```python
from build123d import *

# Parameters (mm, degrees)
SKETCH_1_W          = 33
SKETCH_1_H          = 10
EXTRUDE_1_DEPTH     = 3
HOLE_WIZARD_1_D     = 3.5
SKETCH_5_W          = 33
SKETCH_5_H          = 3
EXTRUDE_2_DEPTH     = 3
SKETCH_6_W          = 33
SKETCH_6_H          = 4
EXTRUDE_3_DEPTH     = 55
SKETCH_7_W          = 50
SKETCH_7_H          = 4
EXTRUDE_4_DEPTH     = 3
SKETCH_8_W          = 50
SKETCH_8_H          = 3
EXTRUDE_5_DEPTH     = 56
EXTRUDE_6_DEPTH     = 5
EXTRUDE_7_DEPTH     = 4
SKETCH_20_W         = 50
SKETCH_20_H         = 3
EXTRUDE_9_DEPTH     = 40
EXTRUDE_15_DEPTH    = 4
EXTRUDE_16_DEPTH    = 4
FILLET_1_R          = 3
HOLE_WIZARD_5_D     = 3.5
HOLE_WIZARD_6_D     = 34
HOLE_WIZARD_7_D     = 2.3
EXTRUDE_17_DEPTH    = 5
SKETCH_49_W         = 44.612037216
SKETCH_49_H         = 28
EXTRUDE_18_DEPTH    = 5
SKETCH_50_W         = 11.25
SKETCH_50_H         = 12
CUT_EXTRUDE_1_DEPTH = 10
EXTRUDE_19_DEPTH    = 5
FILLET_2_R          = 5
SKETCH_52_W         = 3
SKETCH_52_H         = 12
CUT_EXTRUDE_2_DEPTH = 126.136925006
FILLET_3_R          = 3
FILLET_4_R          = 5
SKETCH_53_W         = 5
SKETCH_53_H         = 55.387962784
SKETCH_53_H_2       = 45
EXTRUDE_20_DEPTH    = 4


with BuildPart() as part:
    # 草图1 → 凸台-拉伸1 (new body)
    with BuildSketch(Plane(origin=(0, 0, 0), x_dir=(1, 0, 0), z_dir=(0, 1, 0))):
        Rectangle(SKETCH_1_W, SKETCH_1_H)
    extrude(amount=EXTRUDE_1_DEPTH)

    # 孔1 (through all)
    with Locations(Plane(origin=(0, 3, 0), x_dir=(1, 0, 0), z_dir=(0, 1, 0))):
        with Locations((-13, -1.5), (13, -1.5)):
            Hole(HOLE_WIZARD_1_D / 2)

    # 草图5 → 凸台-拉伸2 (add)
    with BuildSketch(Plane.XZ):
        with Locations((0, -6.5)):
            Rectangle(SKETCH_5_W, SKETCH_5_H)
    extrude(amount=-EXTRUDE_2_DEPTH)

    # 草图6 → 凸台-拉伸3 (add)
    with BuildSketch(Plane(origin=(0, 3, 0), x_dir=(1, 0, 0), z_dir=(0, 1, 0))):
        with Locations((0, 6)):
            Rectangle(SKETCH_6_W, SKETCH_6_H)
    extrude(amount=EXTRUDE_3_DEPTH)

    # 草图7 → 凸台-拉伸4 (add)
    with BuildSketch(Plane(origin=(0, 58, 0), x_dir=(1, 0, 0), z_dir=(0, 1, 0))):
        with Locations((-8.5, 6)):
            Rectangle(SKETCH_7_W, SKETCH_7_H)
    extrude(amount=EXTRUDE_4_DEPTH)

    # 草图8 → 凸台-拉伸5 (add)
    with BuildSketch(Plane(origin=(0, 0, -8), x_dir=(-1, 0, 0), z_dir=(0, 0, -1))):
        with Locations((8.5, 59.5)):
            Rectangle(SKETCH_8_W, SKETCH_8_H)
    extrude(amount=EXTRUDE_5_DEPTH)

    # 草图15 → 凸台-拉伸6 (add)
    with BuildSketch(Plane(origin=(16.5, 0, 0), x_dir=(0, 0, -1), z_dir=(1, 0, 0))):
        Polygon((8, 0), (48.612037216, 58), (42.508164272, 58), (8, 8.717233978), align=None)
    extrude(amount=-EXTRUDE_6_DEPTH)

    # 草图16 → 凸台-拉伸7 (add)
    with BuildSketch(Plane.XY.offset(-4)):
        Polygon((-16.5, 0), (-33.5, 58), (-28.289650608, 58), (-16.5, 17.77648616), align=None)
    extrude(amount=-EXTRUDE_7_DEPTH)

    # 草图20 → 凸台-拉伸9 (add)
    with BuildSketch(Plane(origin=(0, 0, -64), x_dir=(-1, 0, 0), z_dir=(0, 0, -1))):
        with Locations((8.5, 59.5)):
            Rectangle(SKETCH_20_W, SKETCH_20_H)
    extrude(amount=EXTRUDE_9_DEPTH)

    # 草图33 → 凸台-拉伸15 (add)
    with BuildSketch(Plane.XY.offset(-4)):
        Polygon((-28.289650608, 58), (-16.5, 17.77648616), (-16.5, 58), align=None)
    extrude(amount=-EXTRUDE_15_DEPTH)

    # 草图34 → 凸台-拉伸16 (add)
    with BuildSketch(Plane.XY.offset(-4)):
        Polygon((-33.5, 58), (-33.5, 0), (-16.5, 0), align=None)
    extrude(amount=-EXTRUDE_16_DEPTH)

    # 圆角1
    fillet_1_edges = [part.edges().sort_by_distance(p)[0] for p in [
        (-33.5, 0, -6),
    ]]
    fillet(fillet_1_edges, radius=FILLET_1_R)

    # 孔5 (through all)
    with Locations(Plane.XY.offset(-4)):
        with Locations((-24.5, 55), (-24.5, 23), (7.5, 23), (7.5, 55)):
            Hole(HOLE_WIZARD_5_D / 2)

    # 孔6 (through all)
    with Locations(Plane.XY.offset(-4)):
        with Locations((-8.5, 39)):
            Hole(HOLE_WIZARD_6_D / 2)

    # 孔7 (through all)
    with Locations(Plane(origin=(0, 58, 0), x_dir=(-1, 0, 0), z_dir=(0, -1, 0))):
        with Locations((-9, 11), (-9, 47), (27, 47), (27, 11)):
            Hole(HOLE_WIZARD_7_D / 2)

    # 草图48 → 凸台-拉伸17 (add)
    with BuildSketch(Plane(origin=(16.5, 0, 0), x_dir=(0, 0, -1), z_dir=(1, 0, 0))):
        Polygon((8, 8.717233978), (8, 58), (42.508164272, 58), align=None)
    extrude(amount=-EXTRUDE_17_DEPTH)

    # 草图49 → 凸台-拉伸18 (add)
    with BuildSketch(Plane(origin=(16.5, 0, 0), x_dir=(0, 0, -1), z_dir=(1, 0, 0))):
        with Locations((26.306018608, 44)):
            Rectangle(SKETCH_49_W, SKETCH_49_H)
    extrude(amount=-EXTRUDE_18_DEPTH)

    # 草图50 → 切除-拉伸1 (cut)
    with BuildSketch(Plane(origin=(0, 61, 0), x_dir=(1, 0, 0), z_dir=(0, 1, 0))):
        with Locations((5.875, 34)):
            Rectangle(SKETCH_50_W, SKETCH_50_H)
    extrude(amount=-CUT_EXTRUDE_1_DEPTH, mode=Mode.SUBTRACT)

    # 草图51 → 凸台-拉伸19 (add)
    with BuildSketch(Plane(origin=(16.5, 0, 0), x_dir=(0, 0, -1), z_dir=(1, 0, 0))):
        Polygon((29.006226146, 30), (20.967750373, 0), (8, 0), align=None)
    extrude(amount=-EXTRUDE_19_DEPTH)

    # 圆角2
    fillet_2_edges = [part.edges().sort_by_distance(p)[0] for p in [
        (14, 30, -29.006226146),
        (14, 30, -48.612037216),
    ]]
    fillet(fillet_2_edges, radius=FILLET_2_R)

    # 草图52 → 切除-拉伸2 (cut, through all)
    with BuildSketch(Plane(origin=(0, 61, 0), x_dir=(1, 0, 0), z_dir=(0, 1, 0))):
        with Locations((13, 34)):
            Rectangle(SKETCH_52_W, SKETCH_52_H)
    extrude(amount=-CUT_EXTRUDE_2_DEPTH, mode=Mode.SUBTRACT)

    # 圆角3
    fillet_3_edges = [part.edges().sort_by_distance(p)[0] for p in [
        (0.25, 59.5, -28),
        (0.25, 59.5, -40),
        (14.5, 45.5, -40),
        (14.5, 43.622356449, -28),
    ]]
    fillet(fillet_3_edges, radius=FILLET_3_R - 0.0001)  # a hair under: the kernel refuses the full size

    # 圆角4
    fillet_4_edges = [part.edges().sort_by_distance(p)[0] for p in [
        (-16.5, 1.5, -4),
    ]]
    fillet(fillet_4_edges, radius=FILLET_4_R)

    # 草图53 → 凸台-拉伸20 (add)
    with BuildSketch(Plane.XZ.offset(-58)):
        with Locations((14, -76.306018608)):
            Rectangle(SKETCH_53_W, SKETCH_53_H)
        with Locations((-31, -81.5)):
            Rectangle(SKETCH_53_W, SKETCH_53_H_2)
    extrude(amount=EXTRUDE_20_DEPTH)


solid = part.part
```
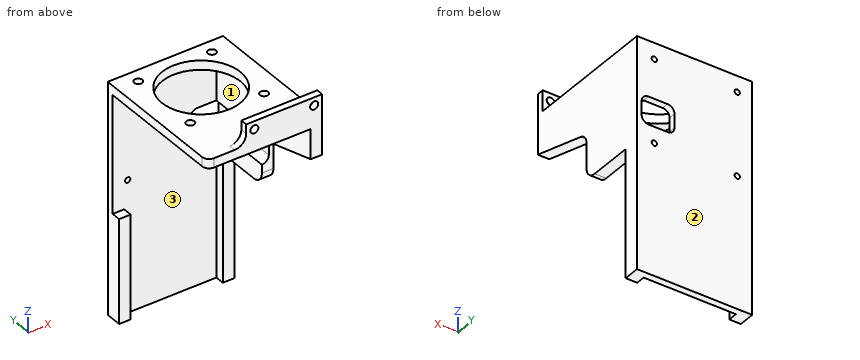
The model under review builds one solid part; all positions refer to its coordinate system, in mm. Face numbers are marked on the shaded views. Give positions to 0.01 mm unless a question says otherwise; leave off trailing zeros. Loops run counter-clockwise (first coordinate to the right, second up) from the corner with the lowest first, then second, coordinate; pieces in that order, holes last. Notation, with made-up numbers: (-13, 74) - (25, 74) arc R22 ccw to (25, 112) - close; hole circle Ø4 at (46.5, 25). An arc over 180 degrees is marked (long way). Answer as a JSON object with one key per item and string values.
Q1. Add section B-B on x = -8.5. State the section outline as (y, z) points.
Worked out:
{"outline": "(0, -8) - (22, -8) - (22, -4) - (3, -4) - (3, 5) - (0, 5) - close; (56, -8) - (58, -8) - (58, -104) - (61, -104) - (61, -4) - (56, -4) - close"}
Q2. Add section A-A on z = -11. State the section outline as (x, y) points.
Worked out:
{"outline": "(-33.5, 58) - (-28.15, 58) - (-28.15, 61) - (-33.5, 61) - close; (-25.85, 58) - (7.85, 58) - (7.85, 61) - (-25.85, 61) - close; (10.15, 58) - (11.5, 58) - (11.5, 0) - (16.5, 0) - (16.5, 61) - (10.15, 61) - close"}
Q3. Insertion check: pin 1 (3 mm diameter, centred on x = 7.5, y = 23, fed in from +Z); pin 2 (4.5 mm diameter, centred on x = -31.5, y = 56, fed in from +Z); pin 3 (9 mm diameter, centred on x = 5.5, y = 45, fed in from -Z); pin 4 (3.5 mm diameter, centred on x = -27, z = -47, fed in from -Y). Each pin has a flat end and moves straight along its axis. Give the tip position at first contact, or say it passes through.
Worked out:
{"pin 1": "passes through", "pin 2": "stops at z = -4", "pin 3": "stops at z = -8", "pin 4": "stops at y = 58"}
Q4. Add section D-D on z = -67. State the section outline as (x, y) points, plus the area to 3 significant figures.
Worked out:
{"outline": "(-33.5, 54) - (-28.5, 54) - (-28.5, 58) - (11.5, 58) - (11.5, 54) - (16.5, 54) - (16.5, 61) - (-33.5, 61) - close", "area": "190 mm^2"}
Q5. Mouldability with a two-part tool opening along X and no side actions: class the marked faces 1, 2 and 3 as +X half, -X half, draft (parallel to the pull), parting line (faces both ways), or undercut.
Worked out:
{"face 1": "-X half", "face 2": "draft", "face 3": "undercut"}
Q6. To check wall thickness, follow line 1 along X through (y, z) = (59.2, -47); line 2 along Z through (x, y) = (9, 58.95); line 3 along Z through (x, y) = (-27, 59.6). State the ranges of each line that lie inside material, in increasing order.
Worked out:
{"line 1": "x = -33.5 to -28.15, -25.85 to 7.85, 10.15 to 16.5", "line 2": "z = -104 to -48.15, -45.85 to -40, -28 to -12.15, -9.85 to -4", "line 3": "z = -104 to -48.15, -45.85 to -12.15, -9.85 to -4"}
